Part model, mm, in its own coordinate system. A direction names the side the tool comes from. Round coordinates to 2 decimals unless told otherwise and drop trailing zeros. Order: outer loops, then holes, each group sorted by start corner. A loop starts at its lowest first (then second) coordinate and runs counter-clockwise, first axis right, second up. Notation, with made-up numbers: (-15, -15) -> (40, -15) arc R13 ccw to (40, -9) -> close; hole circle Ø4 at (-28, -9.75). An arc over 180 degrees is marked (long way). Answer as a JSON object with one key per item and string values. Group by question number.
```python
from build123d import *

# Parameters (mm, degrees)
ESTRUSIONE_ESTRUSIONE1_DEPTH      = 600
ESTRUSIONE_ESTRUSIONE1_DEPTH_BACK = 100
SCHIZZO6_R                        = 30
SCHIZZO7_R                        = 49.111274452
ESTRUSIONE_ESTRUSIONE2_DEPTH      = 10


with BuildPart() as part:
    # Schizzo1 → Rivoluzione2 (revolve)
    with BuildSketch(Plane.XY):
        with BuildLine():
            Line((0, 280.99750454), (0, 300))
            add(Edge.make_bspline(
                [(400, 0), (400, 300), (0, 300)],
                knots=[0, 0, 0, 1.570796327, 1.570796327, 1.570796327], degree=2, weights=[1, 0.707106781, 1]))
            Line((400, 0), (377.926101554, 0))
            add(Edge.make_bspline(
                [(377.926101554, 0), (377.926101554, 280.99750454), (0, 280.99750454)],
                knots=[0, 0, 0, 1.570796327, 1.570796327, 1.570796327], degree=2, weights=[1, 0.707106781, 1]))
        make_face()
    revolve(axis=Axis((0, 300, 0), (0, -1, 0)))

    # Schizzo6 → Estrusione-Estrusione1 (add, two sides: drawn at the far end of the back side and taken through both)
    with BuildSketch(Plane(origin=(0, 0, 0), x_dir=(1, 0, 0), z_dir=(0, 1, 0)).offset(-ESTRUSIONE_ESTRUSIONE1_DEPTH_BACK)):
        with Locations(Location((0, 0, 0), (0, 0, 270))):
            Circle(SCHIZZO6_R)
    extrude(amount=ESTRUSIONE_ESTRUSIONE1_DEPTH + ESTRUSIONE_ESTRUSIONE1_DEPTH_BACK)

    # Schizzo7 → Estrusione-Estrusione2 (add)
    with BuildSketch(Plane.XZ.offset(100)):
        with Locations(Location((0, 0, 0), (0, 0, 270))):
            Circle(SCHIZZO7_R)
    extrude(amount=ESTRUSIONE_ESTRUSIONE2_DEPTH)


solid = part.part
```
Q1. Drop flat-ended pins along their axis: pin 1 Ø5 at (y, z) = (23.5, 182.5) entering from -X; pin 2 Ø12 at (x, z) = (229, -51.5) entering from -Y; pin 3 Ø3 at (y, z) = (190.5, 66.5) entering from -X. Give the stop position or say it passes through.
Q2. Wall check: line 1 (Z direction, x = 24, y = 87); line 2 (Z direction, x = 180, y = 64); line 3 (X direction, y = 179, z = -155). Give the ranges that are in metal, low to high. Write a range as [from, to].
Q3. Which spindle directions (+Z, -Z, +X, -X, +Y, -Y) get a long thin tool onto all of the face, cutting with end or side? Do faces 4 (the flat face through (-21, -100, 23)), 5 (the flat face through (0, 600, 0)), 6 (the cylindrical face through (2.159, -104.93, 49.064)). Say none if no direction does.
Q4. Two-plate mould, pull along Z, no slides. Class faces 1 (the cylindrical face through (1.32, 87.39, -29.97)), 2 (the cylindrical face through (1.32, 447.47, -29.97)), 3 (the flat face through (294, 0, 239)): +Z half, -Z half, draft (parallel to the pull), parting line (faces both ways), or undercut.
Q5. Band-saw the part on A-A (y = 551.5). List the corners of the cut face in (x, z), plus the area to 3 significant figures.
Completed:
{
 "1": {"pin 1": "x = -355.87", "pin 2": "y = 216.62", "pin 3": "x = -303.47"},
 "2": {"line 1": "[-382.06, -358.55], [-18, 18], [358.55, 382.06]", "line 2": "[-346.87, -320.97], [320.97, 346.87]", "line 3": "[-281.09, -246.67], [246.67, 281.09]"},
 "3": {"face 4": "none", "face 5": "+Z, -Z, +X, -X, +Y", "face 6": "-Y"},
 "4": {"face 1": "undercut", "face 2": "parting line", "face 3": "draft"},
 "5": {"outline": "circle Ø60 at (0, 0)", "area": "2,830 mm2"}
}
